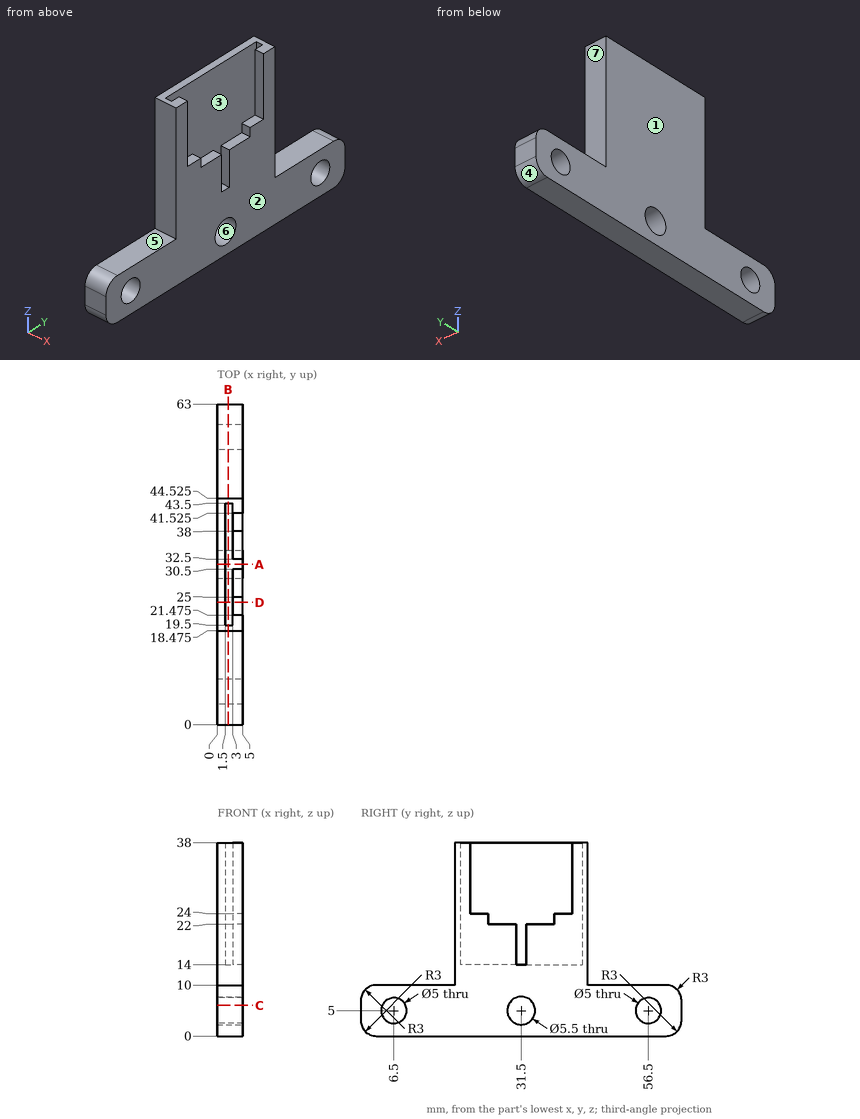
Can you work these out from the drawing? Everything is in mm from the part's minimum corner. A direction names the side the tool comes from. Round coordinates to 2 decimals unless told otherwise and drop trailing zeros. Loops run counter-clockwise (first coordinate to the right, second up) from the corner with the lowest first, then second, coordinate; pieces in that order, holes last. Notation, with made-up numbers: (-16, 65.5) -> (6, 65.5) arc R24 ccw to (6, 90.5) -> close; hole circle Ø6 at (47.25, 4). An arc over 180 degrees is marked (long way). Put each result on its own line as item: value.
Q1. Thinking about a two-plate mould opening in X: for the marked faces 1, 2, 3 and 4, which applies, pulls with the +X half, pulls with the -X half, needs draft (parallel to the pull), parting line crosses it, or undercut?
Checks:
face 1: pulls with the -X half
face 2: pulls with the +X half
face 3: undercut
face 4: needs draft
Q2. I want a section at B-B on x = 2.1. Write out the boundary of the cut face in (y, z) (3 decimals).
Checks:
outline: (0, 3) arc R3 ccw to (3, 0) -> (60, 0) arc R3 ccw to (63, 3) -> (63, 7) arc R3 ccw to (60, 10) -> (44.525, 10) -> (44.525, 38) -> (43.5, 38) -> (43.5, 14) -> (19.5, 14) -> (19.5, 38) -> (18.475, 38) -> (18.475, 10) -> (3, 10) arc R3 ccw to (0, 7) -> close; hole circle Ø5 at (6.5, 5); hole circle Ø5.5 at (31.5, 5); hole circle Ø5 at (56.5, 5)
Q3. I want a section at D-D on y = 24. Write out the boundary of the cut face in (x, z).
Checks:
outline: (0, 0) -> (5, 0) -> (5, 24) -> (3, 24) -> (3, 14) -> (1.5, 14) -> (1.5, 38) -> (0, 38) -> close
Q4. I want a section at A-A on y = 31.5. Write out the boundary of the cut face in (x, z).
Checks:
outline: (0, 0) -> (5, 0) -> (5, 2.25) -> (0, 2.25) -> close; (0, 7.75) -> (5, 7.75) -> (5, 14) -> (1.5, 14) -> (1.5, 38) -> (0, 38) -> close
Q5. For pin 1 Ø1.6 at (x, y) = (4, 28.5) entering from +Z; pin 2 Ø1 at (x, z) = (2, 9.5) entering from +Y; pin 3 Ø4 at (y, z) = (56.5, 5) entering from +X (3 decimals); pin 4 Ø1.6 at (x, z) = (2.5, 30.5) entering from -Y (3 decimals), each with a flat end and sliding along its axis, tell me the tip position at first contact or that it passes through.
Checks:
pin 1: z = 22
pin 2: y = 62.24
pin 3: through
pin 4: y = 18.475
Q6. Which directions (+Z, -Z, +X, -X, +Y, -Y) give clear straight access to the entire face, cutting with the end or side of a thin tool? Please do the marked faces 5, 6 and 7.
Checks:
face 5: +Z, +X, -X, -Y
face 6: +X, -X
face 7: +Z, +X, -X, +Y
Q7. I want a section at C-C on z = 6. Write out the boundary of the cut face in (x, y).
Checks:
outline: (0, 0) -> (5, 0) -> (5, 4.21) -> (0, 4.21) -> close; (0, 8.79) -> (5, 8.79) -> (5, 28.94) -> (0, 28.94) -> close; (0, 34.06) -> (5, 34.06) -> (5, 54.21) -> (0, 54.21) -> close; (0, 58.79) -> (5, 58.79) -> (5, 63) -> (0, 63) -> close
Q8. Please list where these lines run through material, in increasing order: line 1 (Z direction, x = 1.8, y = 31.5); line 2 (Y direction, x = 3.2, z = 16) (3 decimals); line 3 (X direction, y = 25, z = 18). Write a range as from..to.
Checks:
line 1: 0..2.25, 7.75..14
line 2: 18.475..30.5, 32.5..44.525
line 3: 0..1.5, 3..5
